Can you work these out from the model? Positions are in its coordinate system, mm. A direction names the side the tool comes from. Give positions to 0.01 mm unless a question says otherwise; leave off trailing zeros. Write each loop counter-clockwise with the first axis right and the second up, starting at its lowest first coordinate (ties: lowest second). Pieces come first, ordered by that corner, then holes.
```python
from build123d import *

# Parameters (mm, degrees)
SKETCH1_R           = 3.175
BOSS_EXTRUDE1_DEPTH = 9
SKETCH2_R           = 4.75
BOSS_EXTRUDE2_DEPTH = 9.5
SKETCH3_R           = 6.075
BOSS_EXTRUDE3_DEPTH = 4
SKETCH4_R           = 7.05
BOSS_EXTRUDE4_DEPTH = 10
SKETCH5_R           = 7.5
BOSS_EXTRUDE5_DEPTH = 5
SKETCH6_R           = 4.25
BOSS_EXTRUDE6_DEPTH = 3
FILLET1_R           = 3.175


with BuildPart() as part:
    # Sketch1 → Boss-Extrude1 (new body)
    with BuildSketch(Plane.XY):
        Circle(SKETCH1_R)
    extrude(amount=BOSS_EXTRUDE1_DEPTH)

    # Sketch2 → Boss-Extrude2 (add)
    with BuildSketch(Plane(origin=(0, 0, 0), x_dir=(-1, 0, 0), z_dir=(0, 0, -1))):
        Circle(SKETCH2_R)
    extrude(amount=BOSS_EXTRUDE2_DEPTH)

    # Sketch3 → Boss-Extrude3 (add)
    with BuildSketch(Plane(origin=(0, 0, -9.5), x_dir=(-1, 0, 0), z_dir=(0, 0, -1))):
        Circle(SKETCH3_R)
    extrude(amount=BOSS_EXTRUDE3_DEPTH)

    # Sketch4 → Boss-Extrude4 (add)
    with BuildSketch(Plane(origin=(0, 0, -13.5), x_dir=(-1, 0, 0), z_dir=(0, 0, -1))):
        Circle(SKETCH4_R)
    extrude(amount=BOSS_EXTRUDE4_DEPTH)

    # Sketch5 → Boss-Extrude5 (add)
    with BuildSketch(Plane(origin=(0, 0, -23.5), x_dir=(-1, 0, 0), z_dir=(0, 0, -1))):
        Circle(SKETCH5_R)
    extrude(amount=BOSS_EXTRUDE5_DEPTH)

    # Sketch6 → Boss-Extrude6 (add)
    with BuildSketch(Plane(origin=(0, 0, -28.5), x_dir=(-1, 0, 0), z_dir=(0, 0, -1))):
        Circle(SKETCH6_R)
    extrude(amount=BOSS_EXTRUDE6_DEPTH)

    # Fillet1
    fillet1_edges = [part.edges().sort_by_distance(p)[0] for p in [
        (-3.175, 0, 9),
    ]]
    fillet(fillet1_edges, radius=FILLET1_R)


solid = part.part
```
1) For pin 1 Ø5 at (x, z) = (4, -9.5) entering from +Y; pin 2 Ø4 at (x, z) = (2.5, -11) entering from +Y; pin 3 Ø1 at (y, z) = (2.5, -19) entering from -X, each with a flat end and sliding along its axis, tell me the tip position at first contact or that it passes through.
Values follow:
pin 1: stops at y = 5.89
pin 2: stops at y = 6.05
pin 3: stops at x = -6.76
2) Please list where these lines run through material, in increasing order: L1, parallel to Z at x = -2.5, y = 5; L2, parallel to Z at x = -2.5, y = 3.25; L3, parallel to Y at x = 0.25, z = 4.5.
Values follow:
L1: z = -28.5 to -9.5
L2: z = -31.5 to 0
L3: y = -3.17 to 3.17
3) Suppose I cut it at A-A on x = 0. Write out the boundary of the cut face in (y, z) (3 decimals), plus the area to 3 significant figures.
Values follow:
outline: (-7.5, -28.5) - (-4.25, -28.5) - (-4.25, -31.5) - (4.25, -31.5) - (4.25, -28.5) - (7.5, -28.5) - (7.5, -23.5) - (7.05, -23.5) - (7.05, -13.5) - (6.075, -13.5) - (6.075, -9.5) - (4.75, -9.5) - (4.75, 0) - (3.175, 0) - (3.175, 5.825) arc R3.175 ccw to (-3.175, 5.825) - (-3.175, 0) - (-4.75, 0) - (-4.75, -9.5) - (-6.075, -9.5) - (-6.075, -13.5) - (-7.05, -13.5) - (-7.05, -23.5) - (-7.5, -23.5) - close
area: 433 mm2
4) For faces 1 (the face through (-3.253, -6.255, -18.43)), 2 (the face through (-2.285, 3.584, -29.979)), 3 (the face through (7.493, 0.33, -25.965)), which set-ups out of +Z, -Z, +X, -X, +Y, -Y let a thin tool reach every point of the face, with its end or its side?
Values follow:
face 1: +Z
face 2: -Z
face 3: +Z, -Z
5) Suppose I cut it at C-C on z = -1. Write out the boundary of the cut face in (x, y), plus the area to 3 significant figures.
Values follow:
outline: circle Ø9.5 at (0, 0)
area: 70.9 mm2
6) Suppose I cut it at D-D on y = -6.5. Write out the boundary of the cut face in (x, z), plus the area to 3 significant figures.
Values follow:
outline: (-3.74, -28.5) - (3.74, -28.5) - (3.74, -23.5) - (2.73, -23.5) - (2.73, -13.5) - (-2.73, -13.5) - (-2.73, -23.5) - (-3.74, -23.5) - close
area: 92.0 mm2
